Source: CAD feature listing. Evaluate the final solid. Frame: model axes, mm. A direction names the side the tool comes from. Give positions to 0.01 mm unless a question says otherwise; leave off trailing zeros. Write each loop counter-clockwise with the first axis right and the second up, starting at its lowest first coordinate (ties: lowest second). Pieces come first, ordered by that corner, then holes. Notation, with made-up numbers: (82.5, 40.5) - (100.5, 40.5) arc R18 ccw to (100.5, 64.5) - close; hole circle Ø8 at (21.5, 60). An arc over 180 degrees is marked (long way). One line per question, with ' | ' between items. Start each with the question number.
(1) Access query for faces 1 (the flat face through (0, -7.3, 0)), 2 (the flat face through (-1.4, 0, -4.5)), 3 (the flat face through (3, -5.8, 0)). Directions: +Z, -Z, +X, -X, +Y, -Y. A direction counts if a zero-diameter tool reaches every point of the face in a straight line with its end or side. Return the directions, or none.
(2) Pin query (flat end, axial travel): pin 1 (1 mm diameter, centred on x = 4, z = -1.5, fed in from -Y); pin 2 (2 mm diameter, centred on y = -4, z = -1, fed in from +X); pin 3 (4 mm diameter, centred on y = -5, z = -3.5, fed in from +X); pin 4 (1.5 mm diameter, centred on x = 1, y = 4.5, fed in from -Z). Return the tip coordinate at first contact, or that it passes through.
(3) Ray query, line 1 (Y direction, x = -3.25, z = 1.25); line 2 (Y direction, x = 1.25, z = 4.75); line 3 (Z direction, x = 4, y = -4). Return the intervals inside material, ascending. Write a range as [from, to].
(4) Section B-B, the plane z = 0. Return loops of the section in (x, y), plus the area to 3 significant figures.
(5) Section D-D, the plane y = -1.5. Return loops of the section in (x, z), plus the area to 3 significant figures.
(6) Section C-C, the plane y = 1.25. Return loops of the section in (x, z).
(7) Section A-A, the plane x = 0. Return loops of the section in (y, z).
```python
from build123d import *

# Parameters (mm, degrees)
SKETCH1_R           = 6
BOSS_EXTRUDE2_DEPTH = 5.8
SKETCH5_R           = 4.5
BOSS_EXTRUDE3_DEPTH = 7
SKETCH6_R           = 2.5
BOSS_EXTRUDE4_DEPTH = 1.5


with BuildPart() as part:
    # Sketch1 → Boss-Extrude2 (new body)
    with BuildSketch(Plane(origin=(0, 0, 0), x_dir=(1, 0, 0), z_dir=(0, 1, 0))):
        Circle(SKETCH1_R)
    extrude(amount=-BOSS_EXTRUDE2_DEPTH)

    # Sketch5 → Boss-Extrude3 (add)
    with BuildSketch(Plane(origin=(0, 0, 0), x_dir=(-1, 0, 0), z_dir=(0, 1, 0))):
        Circle(SKETCH5_R)
    extrude(amount=BOSS_EXTRUDE3_DEPTH)

    # Sketch6 → Boss-Extrude4 (add)
    with BuildSketch(Plane.XZ.offset(5.8)):
        Circle(SKETCH6_R)
    extrude(amount=BOSS_EXTRUDE4_DEPTH)


solid = part.part
```
Check sheet entries:
1) face 1: +Z, -Z, +X, -X, -Y | face 2: +Y | face 3: -Y
2) pin 1: y = -5.8 | pin 2: x = 6 | pin 3: x = 5.81 | pin 4: z = -4.49
3) line 1: [-5.8, 7] | line 2: [-5.8, 0] | line 3: [-4.47, 4.47]
4) outline: (-6, -5.8) - (-2.5, -5.8) - (-2.5, -7.3) - (2.5, -7.3) - (2.5, -5.8) - (6, -5.8) - (6, 0) - (4.5, 0) - (4.5, 7) - (-4.5, 7) - (-4.5, 0) - (-6, 0) - close | area: 140 mm²
5) outline: circle Ø12 at (0, 0) | area: 113 mm²
6) outline: circle Ø9 at (0, 0)
7) outline: (-7.3, -2.5) - (-5.8, -2.5) - (-5.8, -6) - (0, -6) - (0, -4.5) - (7, -4.5) - (7, 4.5) - (0, 4.5) - (0, 6) - (-5.8, 6) - (-5.8, 2.5) - (-7.3, 2.5) - close
